Verification items for the finished model (mm, model axes). Face numbers are marked on the shaded views. A direction names the side the tool comes from. Give positions to 0.01 mm unless a question says otherwise; leave off trailing zeros. Loops run counter-clockwise (first coordinate to the right, second up) from the corner with the lowest first, then second, coordinate; pieces in that order, holes last. Notation, with made-up numbers: (-24, 4) - (26, 4) arc R24 cw to (26, 32) - close; hole circle Ø7 at (51.5, -17.5). An arc over 180 degrees is marked (long way). Use one line per item in the form item = value.
```python
from build123d import *

# Parameters (mm, degrees)
F0_R      = 9.525
F1_DEPTH  = 1.5875
F2_R      = 7.8994
F3_DEPTH  = 3.175
F4_R      = 4.953
F5_DEPTH  = 3.175
F6_R      = 1.7272
F7_DEPTH  = 1.5885
F8_R      = 4.7625
F8_R_2    = 1.7272
F9_DEPTH  = 6.35
F10_R     = 3.2131
F11_DEPTH = 3.175
F12_R     = 4.064
F13_DEPTH = 3.71856


with BuildPart() as f1:
    # F0 (on Top) → F1 (new body)
    with BuildSketch(Plane.XY):
        Circle(F0_R)
    extrude(amount=F1_DEPTH)

    # F2 (on face) → F3 (join)
    with BuildSketch(Plane.XY.offset(1.5875)):
        Circle(F2_R)
    extrude(amount=F3_DEPTH)

    # F4 (on face) → F5 (cut)
    with BuildSketch(Plane(origin=(0, 0, 0), x_dir=(1, 0, 0), z_dir=(0, 0, -1))):
        Circle(F4_R)
    extrude(amount=-F5_DEPTH, mode=Mode.SUBTRACT)

    # F6 (on face) → F7 (cut, through all)
    with BuildSketch(Plane(origin=(0, 0, 3.175), x_dir=(1, 0, 0), z_dir=(0, 0, -1))):
        Circle(F6_R)
    extrude(amount=-F7_DEPTH, mode=Mode.SUBTRACT)

    # F8 (on face) → F9 (join)
    with BuildSketch(Plane.XY.offset(4.7625)):
        Circle(F8_R)
        Circle(F8_R_2, mode=Mode.SUBTRACT)
    extrude(amount=F9_DEPTH)

    # F10 (on face) → F11 (cut)
    with BuildSketch(Plane.XY.offset(11.1125)):
        Circle(F10_R)
    extrude(amount=-F11_DEPTH, mode=Mode.SUBTRACT)

    # F12 (on face) → F13 (cut)
    with BuildSketch(Plane(origin=(0, 0, 3.175), x_dir=(1, 0, 0), z_dir=(0, 0, -1))):
        Circle(F12_R)
    extrude(amount=-F13_DEPTH, mode=Mode.SUBTRACT)


solid = f1.part
```
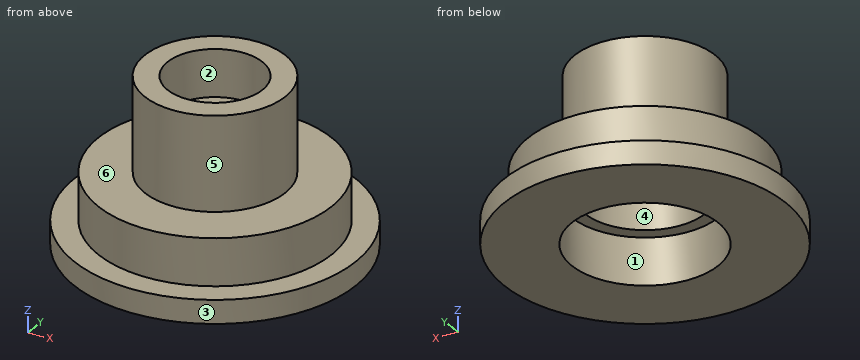
1. Section check C-C, the plane z = 10.25. Record the cut outline in (x, y) (1 decimal), then the cut area to 3 significant figures.
Result set:
outline = circle Ø9.5 at (0, 0); hole circle Ø6.4 at (0, 0)
area = 38.8 mm²
2. Draft check along Y on the marked faces 4, 5 and 6. Enter one of: released by +Y, released by -Y, zero draft, split by the parting line, or undercut.
Result set:
face_4 = undercut
face_5 = split by the parting line
face_6 = zero draft
3. Depth check by flat-ended pin: pin 1 Ø6 at (y, z) = (1, 5.5) entering from -X; pin 2 Ø6 at (x, y) = (0, 0) entering from +Z; pin 3 Ø5 at (x, y) = (0, 0) entering from -Z; pin 4 Ø1 at (x, z) = (-6, 5.5) entering from +Y. Enter the tip coordinate at first touch or a pass-through.
Result set:
pin_1 = -7.9
pin_2 = 7.94
pin_3 = 6.89
pin_4 = through
4. Section check A-A, the plane x = 0. Record the cut outline in (y, z) (1 decimal), then the cut area to 3 significant figures.
Result set:
outline = (-9.5, 0) - (-5, 0) - (-5, 3.2) - (-4.1, 3.2) - (-4.1, 6.9) - (-1.7, 6.9) - (-1.7, 7.9) - (-3.2, 7.9) - (-3.2, 11.1) - (-4.8, 11.1) - (-4.8, 4.8) - (-7.9, 4.8) - (-7.9, 1.6) - (-9.5, 1.6) - close; (1.7, 6.9) - (4.1, 6.9) - (4.1, 3.2) - (5, 3.2) - (5, 0) - (9.5, 0) - (9.5, 1.6) - (7.9, 1.6) - (7.9, 4.8) - (4.8, 4.8) - (4.8, 11.1) - (3.2, 11.1) - (3.2, 7.9) - (1.7, 7.9) - close
area = 55.2 mm²
5. Scan lines: probe 1 along Y at (x, z) = (0, 5.15); probe 2 along Z at (x, y) = (-5, -1.5); probe 3 along Y at (x, z) = (0, 4.25). Record each from-to range of solid material in increasing order.
Result set:
probe_1 = -4.76 to -4.06, 4.06 to 4.76
probe_2 = 0 to 4.76
probe_3 = -7.9 to -4.06, 4.06 to 7.9
6. Tool access check on the marked faces 1, 2 and 3. Record the directions out of +Z, -Z, +X, -X, +Y, -Y that give a thin tool (end or side, any length) a straight path to the whole face; none if there is none.
Result set:
face_1 = -Z
face_2 = +Z
face_3 = +Z, -Z
7. Section check D-D, the plane y = -7.5. Record the cut outline in (x, z).
Result set:
outline = (-5.87, 0) - (5.87, 0) - (5.87, 1.59) - (2.48, 1.59) - (2.48, 4.76) - (-2.48, 4.76) - (-2.48, 1.59) - (-5.87, 1.59) - close
